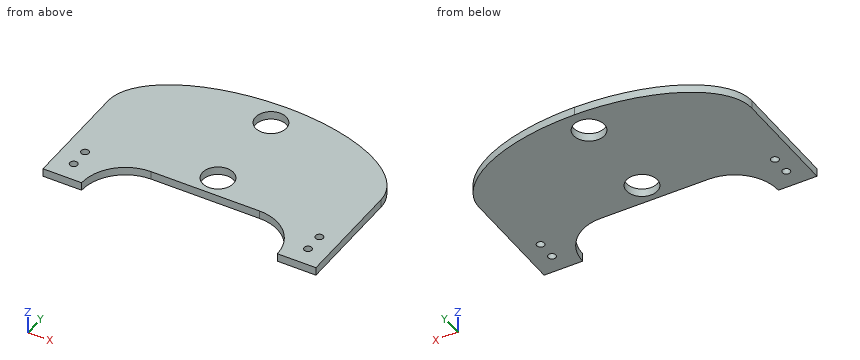
```python
from build123d import *

# Parameters (mm, degrees)
SKETCH1_R           = 6
BOSS_EXTRUDE1_DEPTH = 3.175
SKETCH4_R           = 1.5
CUT_EXTRUDE2_DEPTH  = 128.067228761
CUT_EXTRUDE4_DEPTH  = 128.067228761


with BuildPart() as part:
    # Sketch1 → Boss-Extrude1 (new body)
    with BuildSketch(Plane.XY):
        with BuildLine():
            ThreePointArc((15, 0), (19.97918472, 12.02081528), (32, 17))
            Line((32, 17), (53, 17))
            Line((53, 17), (74, 17))
            ThreePointArc((74, 17), (86.02081528, 12.02081528), (91, 0))
            Line((91, 0), (106, 0))
            Line((106, 0), (106, 70))
            Line((106, 70), (0, 70))
            Line((0, 70), (0, 0))
            Line((0, 0), (15, 0))
        make_face()
        with Locations((53, 25.4)):
            Circle(SKETCH1_R, mode=Mode.SUBTRACT)
        with Locations((53, 60.325)):
            Circle(SKETCH1_R, mode=Mode.SUBTRACT)
    extrude(amount=BOSS_EXTRUDE1_DEPTH)

    # Sketch4 → Cut-Extrude2 (cut, through all)
    with BuildSketch(Plane(origin=(0, 0, 0), x_dir=(-1, 0, 0), z_dir=(0, 0, -1))):
        with Locations((-7.5, 15)):
            Circle(SKETCH4_R)
        with Locations((-7.5, 7.5)):
            Circle(SKETCH4_R)
        with Locations((-98.5, 7.5)):
            Circle(SKETCH4_R)
        with Locations((-98.5, 15)):
            Circle(SKETCH4_R)
    extrude(amount=-CUT_EXTRUDE2_DEPTH, mode=Mode.SUBTRACT)

    # Sketch6 → Cut-Extrude4 (cut, through all)
    with BuildSketch(Plane(origin=(0, 0, 0), x_dir=(-1, 0, 0), z_dir=(0, 0, -1))):
        with BuildLine():
            add(Edge.make_bspline(
                [(-53, 70), (-106, 70), (-106, 42.8625)],
                knots=[1.570796327, 1.570796327, 1.570796327, 3.141592654, 3.141592654, 3.141592654], degree=2, weights=[1, 0.707106781, 1]))
            Line((-53, 70), (-106, 70))
            Line((-106, 70), (-106, 42.8625))
        make_face()
        with BuildLine():
            add(Edge.make_bspline(
                [(0, 42.8625), (0, 70), (-53, 70)],
                knots=[0, 0, 0, 1.570796327, 1.570796327, 1.570796327], degree=2, weights=[1, 0.707106781, 1]))
            Line((0, 42.8625), (0, 70))
            Line((0, 70), (-53, 70))
        make_face()
    extrude(amount=-CUT_EXTRUDE4_DEPTH, mode=Mode.SUBTRACT)


solid = part.part
```
Work out the finished part from the listing and answer in its coordinate system (mm). Give positions to 0.01 mm unless a question says otherwise; leave off trailing zeros. Loops run counter-clockwise (first coordinate to the right, second up) from the corner with the lowest first, then second, coordinate; pieces in that order, holes last. Notation, with made-up numbers: (0, 88.25) - (43, 88.25) arc R8 cw to (43, 99.25) - close; hole circle Ø4 at (14, 52.25). An arc over 180 degrees is marked (long way). Use CSV: the item, a comma, the result in double quotes. Start each with the question number.
(1) Find section C-C, the plane z = 0.7. Count the separate pieces of the cut face and the enclosed holes in it, plus the area to 3 significant figures.
(2) Find section B-B, the plane y = 15. Determine the outline of the cut face in (x, z) (3 decimals).
(3) Each of these flat-tipped pins is pushed along its axis until it touches: pin 1 (5 mm diameter, centred on x = 7.5, y = 7.5, fed in from -Z); pin 2 (2.5 mm diameter, centred on x = 98.5, y = 7.5, fed in from -Z); pin 3 (1.5 mm diameter, centred on y = 49.5, z = 2.5, fed in from -X). Where does it stop, or does it pass through?
(4) Find the intervals of material crossed by L1, parallel to Y at x = 98.5, z = 1.8; L2, parallel to Y at x = 97.5, z = 2.75; L3, parallel to X at y = 25, z = 0.6, in increasing order.
(5) Find section A-A, the plane y = 25.4. Determine the outline of the cut face in (x, z) (3 decimals), plus the area to 3 significant figures.
Results found:
1,separate pieces,"1"
1,enclosed holes,"6"
1,area,"5,380 mm^2"
2,outline,"(0, 0) - (6, 0) - (6, 3.175) - (0, 3.175) - close; (9, 0) - (24, 0) - (24, 3.175) - (9, 3.175) - close; (82, 0) - (97, 0) - (97, 3.175) - (82, 3.175) - close; (100, 0) - (106, 0) - (106, 3.175) - (100, 3.175) - close"
3,pin 1,"z = 0"
3,pin 2,"through"
3,pin 3,"x = 1.26"
4,L1,"0 to 6, 9 to 13.5, 16.5 to 56.78"
4,L2,"0 to 6.38, 8.62 to 13.88, 16.12 to 57.6"
4,L3,"0 to 47.01, 58.99 to 106"
5,outline,"(0, 0) - (47, 0) - (47, 3.175) - (0, 3.175) - close; (59, 0) - (106, 0) - (106, 3.175) - (59, 3.175) - close"
5,area,"298 mm^2"
